```python
from build123d import *

# Parameters (mm, degrees)
SKETCH_1_R      = 2.55
EXTRUDE_1_DEPTH = 200


with BuildPart() as part:
    # 草图1 → 凸台-拉伸1 (new body)
    with BuildSketch(Plane(origin=(0, 0, 0), x_dir=(1, 0, 0), z_dir=(0, 1, 0))):
        with BuildLine():
            Line((19.761209246, 22.533499136), (19.761209246, 21.633499136))
            ThreePointArc((19.761209246, 21.633499136), (19.702630602, 21.49207778), (19.561209246, 21.433499136))
            Line((19.561209246, 21.433499136), (17.861209246, 21.433499136))
            ThreePointArc((17.861209246, 21.433499136), (17.507655855, 21.287052526), (17.361209246, 20.933499136))
            Line((17.361209246, 20.933499136), (17.361209246, 20.001266089))
            ThreePointArc((17.361209246, 20.001266089), (17.39926948, 19.809924373), (17.507655855, 19.647712698))
            Line((17.507655855, 19.647712698), (19.728976199, 17.426392355))
            ThreePointArc((19.728976199, 17.426392355), (20.053399548, 17.209619603), (20.43608298, 17.133499136))
            Line((20.43608298, 17.133499136), (25.286335512, 17.133499136))
            ThreePointArc((25.286335512, 17.133499136), (25.669018944, 17.209619603), (25.993442293, 17.426392355))
            Line((25.993442293, 17.426392355), (28.214762636, 19.647712698))
            ThreePointArc((28.214762636, 19.647712698), (28.323149012, 19.809924373), (28.361209246, 20.001266089))
            Line((28.361209246, 20.001266089), (28.361209246, 20.933499136))
            ThreePointArc((28.361209246, 20.933499136), (28.214762636, 21.287052526), (27.861209246, 21.433499136))
            Line((27.861209246, 21.433499136), (26.161209246, 21.433499136))
            ThreePointArc((26.161209246, 21.433499136), (26.01978789, 21.49207778), (25.961209246, 21.633499136))
            Line((25.961209246, 21.633499136), (25.961209246, 22.533499136))
            ThreePointArc((25.961209246, 22.533499136), (26.01978789, 22.674920492), (26.161209246, 22.733499136))
            Line((26.161209246, 22.733499136), (26.311209246, 22.733499136))
            ThreePointArc((26.311209246, 22.733499136), (26.452630602, 22.79207778), (26.511209246, 22.933499136))
            Line((26.511209246, 22.933499136), (26.511209246, 23.033499136))
            ThreePointArc((26.511209246, 23.033499136), (26.56978789, 23.174920492), (26.711209246, 23.233499136))
            Line((26.711209246, 23.233499136), (31.361209246, 23.233499136))
            ThreePointArc((31.361209246, 23.233499136), (32.421869418, 22.794159308), (32.861209246, 21.733499136))
            Line((32.861209246, 21.733499136), (32.861209246, 17.083499136))
            ThreePointArc((32.861209246, 17.083499136), (32.802630602, 16.94207778), (32.661209246, 16.883499136))
            Line((32.661209246, 16.883499136), (32.561209246, 16.883499136))
            ThreePointArc((32.561209246, 16.883499136), (32.41978789, 16.824920492), (32.361209246, 16.683499136))
            Line((32.361209246, 16.683499136), (32.361209246, 16.533499136))
            ThreePointArc((32.361209246, 16.533499136), (32.302630602, 16.39207778), (32.161209246, 16.333499136))
            Line((32.161209246, 16.333499136), (31.261209246, 16.333499136))
            ThreePointArc((31.261209246, 16.333499136), (31.11978789, 16.39207778), (31.061209246, 16.533499136))
            Line((31.061209246, 16.533499136), (31.061209246, 18.233499136))
            ThreePointArc((31.061209246, 18.233499136), (30.914762636, 18.587052526), (30.561209246, 18.733499136))
            Line((30.561209246, 18.733499136), (29.628976199, 18.733499136))
            ThreePointArc((29.628976199, 18.733499136), (29.437634483, 18.695438902), (29.275422808, 18.587052526))
            Line((29.275422808, 18.587052526), (27.054102465, 16.365732183))
            ThreePointArc((27.054102465, 16.365732183), (26.837329713, 16.041308834), (26.761209246, 15.658625402))
            Line((26.761209246, 15.658625402), (26.761209246, 10.80837287))
            ThreePointArc((26.761209246, 10.80837287), (26.837329713, 10.425689438), (27.054102465, 10.101266089))
            Line((27.054102465, 10.101266089), (29.275422808, 7.879945745))
            ThreePointArc((29.275422808, 7.879945745), (29.437634483, 7.77155937), (29.628976199, 7.733499136))
            Line((29.628976199, 7.733499136), (30.561209246, 7.733499136))
            ThreePointArc((30.561209246, 7.733499136), (30.914762636, 7.879945745), (31.061209246, 8.233499136))
            Line((31.061209246, 8.233499136), (31.061209246, 9.933499136))
            ThreePointArc((31.061209246, 9.933499136), (31.11978789, 10.074920492), (31.261209246, 10.133499136))
            Line((31.261209246, 10.133499136), (32.161209246, 10.133499136))
            ThreePointArc((32.161209246, 10.133499136), (32.302630602, 10.074920492), (32.361209246, 9.933499136))
            Line((32.361209246, 9.933499136), (32.361209246, 9.783499136))
            ThreePointArc((32.361209246, 9.783499136), (32.41978789, 9.64207778), (32.561209246, 9.583499136))
            Line((32.561209246, 9.583499136), (32.661209246, 9.583499136))
            ThreePointArc((32.661209246, 9.583499136), (32.802630602, 9.524920492), (32.861209246, 9.383499136))
            Line((32.861209246, 9.383499136), (32.861209246, 4.733499136))
            ThreePointArc((32.861209246, 4.733499136), (32.421869418, 3.672838964), (31.361209246, 3.233499136))
            Line((31.361209246, 3.233499136), (26.711209246, 3.233499136))
            ThreePointArc((26.711209246, 3.233499136), (26.56978789, 3.29207778), (26.511209246, 3.433499136))
            Line((26.511209246, 3.433499136), (26.511209246, 3.533499136))
            ThreePointArc((26.511209246, 3.533499136), (26.452630602, 3.674920492), (26.311209246, 3.733499136))
            Line((26.311209246, 3.733499136), (26.161209246, 3.733499136))
            ThreePointArc((26.161209246, 3.733499136), (26.01978789, 3.79207778), (25.961209246, 3.933499136))
            Line((25.961209246, 3.933499136), (25.961209246, 4.833499136))
            ThreePointArc((25.961209246, 4.833499136), (26.01978789, 4.974920492), (26.161209246, 5.033499136))
            Line((26.161209246, 5.033499136), (27.861209246, 5.033499136))
            ThreePointArc((27.861209246, 5.033499136), (28.214762636, 5.179945745), (28.361209246, 5.533499136))
            Line((28.361209246, 5.533499136), (28.361209246, 6.465732183))
            ThreePointArc((28.361209246, 6.465732183), (28.323149012, 6.657073899), (28.214762636, 6.819285573))
            Line((28.214762636, 6.819285573), (25.993442293, 9.040605917))
            ThreePointArc((25.993442293, 9.040605917), (25.669018944, 9.257378668), (25.286335512, 9.333499136))
            Line((25.286335512, 9.333499136), (20.43608298, 9.333499136))
            ThreePointArc((20.43608298, 9.333499136), (20.053399548, 9.257378668), (19.728976199, 9.040605917))
            Line((19.728976199, 9.040605917), (17.507655855, 6.819285573))
            ThreePointArc((17.507655855, 6.819285573), (17.39926948, 6.657073899), (17.361209246, 6.465732183))
            Line((17.361209246, 6.465732183), (17.361209246, 5.533499136))
            ThreePointArc((17.361209246, 5.533499136), (17.507655855, 5.179945745), (17.861209246, 5.033499136))
            Line((17.861209246, 5.033499136), (19.561209246, 5.033499136))
            ThreePointArc((19.561209246, 5.033499136), (19.702630602, 4.974920492), (19.761209246, 4.833499136))
            Line((19.761209246, 4.833499136), (19.761209246, 3.933499136))
            ThreePointArc((19.761209246, 3.933499136), (19.702630602, 3.79207778), (19.561209246, 3.733499136))
            Line((19.561209246, 3.733499136), (19.411209246, 3.733499136))
            ThreePointArc((19.411209246, 3.733499136), (19.26978789, 3.674920492), (19.211209246, 3.533499136))
            Line((19.211209246, 3.533499136), (19.211209246, 3.433499136))
            ThreePointArc((19.211209246, 3.433499136), (19.152630602, 3.29207778), (19.011209246, 3.233499136))
            Line((19.011209246, 3.233499136), (14.361209246, 3.233499136))
            ThreePointArc((14.361209246, 3.233499136), (13.300549074, 3.672838964), (12.861209246, 4.733499136))
            Line((12.861209246, 4.733499136), (12.861209246, 9.383499136))
            ThreePointArc((12.861209246, 9.383499136), (12.91978789, 9.524920492), (13.061209246, 9.583499136))
            Line((13.061209246, 9.583499136), (13.161209246, 9.583499136))
            ThreePointArc((13.161209246, 9.583499136), (13.302630602, 9.64207778), (13.361209246, 9.783499136))
            Line((13.361209246, 9.783499136), (13.361209246, 9.933499136))
            ThreePointArc((13.361209246, 9.933499136), (13.41978789, 10.074920492), (13.561209246, 10.133499136))
            Line((13.561209246, 10.133499136), (14.461209246, 10.133499136))
            ThreePointArc((14.461209246, 10.133499136), (14.602630602, 10.074920492), (14.661209246, 9.933499136))
            Line((14.661209246, 9.933499136), (14.661209246, 8.233499136))
            ThreePointArc((14.661209246, 8.233499136), (14.807655855, 7.879945745), (15.161209246, 7.733499136))
            Line((15.161209246, 7.733499136), (16.093442293, 7.733499136))
            ThreePointArc((16.093442293, 7.733499136), (16.284784009, 7.77155937), (16.446995684, 7.879945745))
            Line((16.446995684, 7.879945745), (18.668316027, 10.101266089))
            ThreePointArc((18.668316027, 10.101266089), (18.885088778, 10.425689438), (18.961209246, 10.80837287))
            Line((18.961209246, 10.80837287), (18.961209246, 13.233499136))
            Line((18.961209246, 13.233499136), (18.961209246, 15.658625402))
            ThreePointArc((18.961209246, 15.658625402), (18.885088778, 16.041308834), (18.668316027, 16.365732183))
            Line((18.668316027, 16.365732183), (16.446995684, 18.587052526))
            ThreePointArc((16.446995684, 18.587052526), (16.284784009, 18.695438902), (16.093442293, 18.733499136))
            Line((16.093442293, 18.733499136), (15.161209246, 18.733499136))
            ThreePointArc((15.161209246, 18.733499136), (14.807655855, 18.587052526), (14.661209246, 18.233499136))
            Line((14.661209246, 18.233499136), (14.661209246, 16.533499136))
            ThreePointArc((14.661209246, 16.533499136), (14.602630602, 16.39207778), (14.461209246, 16.333499136))
            Line((14.461209246, 16.333499136), (13.561209246, 16.333499136))
            ThreePointArc((13.561209246, 16.333499136), (13.41978789, 16.39207778), (13.361209246, 16.533499136))
            Line((13.361209246, 16.533499136), (13.361209246, 16.683499136))
            ThreePointArc((13.361209246, 16.683499136), (13.302630602, 16.824920492), (13.161209246, 16.883499136))
            Line((13.161209246, 16.883499136), (13.061209246, 16.883499136))
            ThreePointArc((13.061209246, 16.883499136), (12.91978789, 16.94207778), (12.861209246, 17.083499136))
            Line((12.861209246, 17.083499136), (12.861209246, 21.733499136))
            ThreePointArc((12.861209246, 21.733499136), (13.300549074, 22.794159308), (14.361209246, 23.233499136))
            Line((14.361209246, 23.233499136), (19.011209246, 23.233499136))
            ThreePointArc((19.011209246, 23.233499136), (19.152630602, 23.174920492), (19.211209246, 23.033499136))
            Line((19.211209246, 23.033499136), (19.211209246, 22.933499136))
            ThreePointArc((19.211209246, 22.933499136), (19.26978789, 22.79207778), (19.411209246, 22.733499136))
            Line((19.411209246, 22.733499136), (19.561209246, 22.733499136))
            ThreePointArc((19.561209246, 22.733499136), (19.702630602, 22.674920492), (19.761209246, 22.533499136))
        make_face()
        with Locations(Location((22.861209246, 13.233499136, 0), (0, 0, 270))):
            Circle(SKETCH_1_R, mode=Mode.SUBTRACT)
    extrude(amount=EXTRUDE_1_DEPTH)


solid = part.part
```
Here's how the part is built. I have some questions about the finished solid (model axes, mm). A direction names the side the tool comes from. Coordinates: 2 decimals unless noted, no trailing zeros. Order: outer loops, then holes, each group sorted by start corner. A loop starts at its lowest first (then second) coordinate and runs counter-clockwise, first axis right, second up.
Item 1: Which directions (+Z, -Z, +X, -X, +Y, -Y) give clear straight access to the entire face, cutting with the end or side of a thin tool? Please do faces 1 (the face through (18.961, 99, -13)), 2 (the face through (23, 99, -17.133)), 3 (the face through (23, 99, -9.333)).
Response values:
face 1: -X, +Y, -Y
face 2: -Z, +Y, -Y
face 3: +Z, +Y, -Y
Item 2: I'm going to push flat-ended pins straight in: pin 1 Ø1.5 at (x, y) = (24, 74.5) entering from +Z; pin 2 Ø3 at (x, y) = (21, 143) entering from +Z. Where does each tip first touch, or does it pass through?
Response values:
pin 1: stops at z = -9.33
pin 2: stops at z = -3.73
Item 3: If we section it at A-A, the plane z = -14: List the corners of the cut face in (x, y) for me, then the cut area to 3 significant figures.
Response values:
outline: (18.96, 0) - (20.43, 0) - (20.43, 200) - (18.96, 200) - close; (25.29, 0) - (26.76, 0) - (26.76, 200) - (25.29, 200) - close
area: 587 mm2
Item 4: I need wall thicknesses on probe 1 along Z at (x, y) = (23.75, 42); probe 2 along Z at (x, y) = (30.75, 58); probe 3 along X at (y, z) = (20, -20.5). Which ranges of each line are inside material? Lowest first, please.
Response values:
probe 1: z = -17.13 to -15.62, -10.84 to -9.33
probe 2: z = -23.23 to -18.7, -7.77 to -3.23
probe 3: x = 12.86 to 17.36, 28.36 to 32.86
Item 5: Thinking about a two-plate mould opening in Z: for faces 4 (the face through (32.861, 99, -19)), 5 (the face through (29, 99, -3.233)), 6 (the face through (22.97, 98.6, -15.78)), which applies, pulls with the +Z half, pulls with the -Z half, needs draft (parallel to the pull), parting line crosses it, or undercut?
Response values:
face 4: needs draft
face 5: pulls with the +Z half
face 6: undercut
